For this review, take the finished solid that the model builds, in its own axes (mm). Face numbers are marked on the shaded views. A direction names the side the tool comes from. Coordinates: 2 decimals unless noted, no trailing zeros. Write each loop counter-clockwise with the first axis right and the second up, starting at its lowest first coordinate (ties: lowest second). Pieces come first, ordered by that corner, then holes. Notation, with made-up numbers: (72.25, 67.25) -> (115.25, 67.25) arc R17 ccw to (115.25, 84.25) -> close; hole circle Ø10 at (26.5, 21.25). An arc over 180 degrees is marked (long way). One line per item, written item: value. Start each with the question number.
1) Mouldability with a two-part tool opening along Z and no side actions: class the marked faces 3, 4 and 5 as released by +Z, released by -Z, zero draft, split by the parting line, or undercut.
2) Add section A-A (x = -10). State the section outline as (y, z) points.
3) Add section B-B (y = 15). State the section outline as (x, z) points.
4) For probe 1 along Y at (x, z) = (-20, 24.25); probe 2 along Z at (x, y) = (-3, 53); probe 3 along X at (y, z) = (41.5, 4.5), list the stretches that pass through material, from the lowest coordinate up. Write a range as from..to.
5) Add section D-D (y = 5.5). State the section outline as (x, z) points, and give its area (3 significant figures).
6) For pin 1 Ø6 at (x, z) = (-5, 19.5) entering from +Y; pin 2 Ø2 at (y, z) = (64.5, -8.5) entering from +X, all flat-tipped, find the tip position at first contact; note any pin that passes through.
7) Add section C-C (x = -20). State the section outline as (y, z) points, and give its area (3 significant figures).
8) Machinability: for the marked faces 1 and 2, which of the approach directions +Z, -Z, +X, -X, +Y, -Y give a long, thin tool a straight path to every point of the face, cutting with its end or side? Answer none if there is none.
from build123d import *

# Parameters (mm, degrees)
SKETCH_1_W          = 74
SKETCH_1_H          = 44
EXTRUDE_1_DEPTH     = 80
SKETCH_2_W          = 41.146480438
SKETCH_2_H          = 58.393385187
CUT_EXTRUDE_1_DEPTH = 81
SKETCH_3_R          = 4.05
CUT_EXTRUDE_2_DEPTH = 51


with BuildPart() as part:
    # Эскиз1 → Вытянуть-Тонкостенный1 (new body)
    with BuildSketch(Plane(origin=(0, 0, 0), x_dir=(1, 0, 0), z_dir=(0, 1, 0))):
        with BuildLine():
            Line((40, 22), (40, -22))
            ThreePointArc((40, -22), (39.121320344, -24.121320344), (37, -25))
            Line((37, -25), (-37, -25))
            ThreePointArc((-37, -25), (-39.121320344, -24.121320344), (-40, -22))
            Line((-40, -22), (-40, 22))
            ThreePointArc((-40, 22), (-39.121320344, 24.121320344), (-37, 25))
            Line((-37, 25), (37, 25))
            ThreePointArc((37, 25), (39.121320344, 24.121320344), (40, 22))
        make_face()
        Rectangle(SKETCH_1_W, SKETCH_1_H, mode=Mode.SUBTRACT)
    extrude(amount=EXTRUDE_1_DEPTH)

    # Эскиз2 → Вырез-Вытянуть1 (cut, through all)
    with BuildSketch(Plane(origin=(0, 80, 0), x_dir=(1, 0, 0), z_dir=(0, 1, 0))):
        with Locations((20.573240219, 1.776081122)):
            Rectangle(SKETCH_2_W, SKETCH_2_H)
    extrude(amount=-CUT_EXTRUDE_1_DEPTH, mode=Mode.SUBTRACT)

    # Эскиз3 → Вырез-Вытянуть2 (cut, through all)
    with BuildSketch(Plane(origin=(0, 0, -25), x_dir=(-1, 0, 0), z_dir=(0, 0, -1))):
        with Locations((20, 115)):
            Circle(SKETCH_3_R)
        with Locations((20, 15)):
            Circle(SKETCH_3_R)
        with Locations((20, 65)):
            Circle(SKETCH_3_R)
    extrude(amount=-CUT_EXTRUDE_2_DEPTH, mode=Mode.SUBTRACT)


solid = part.part
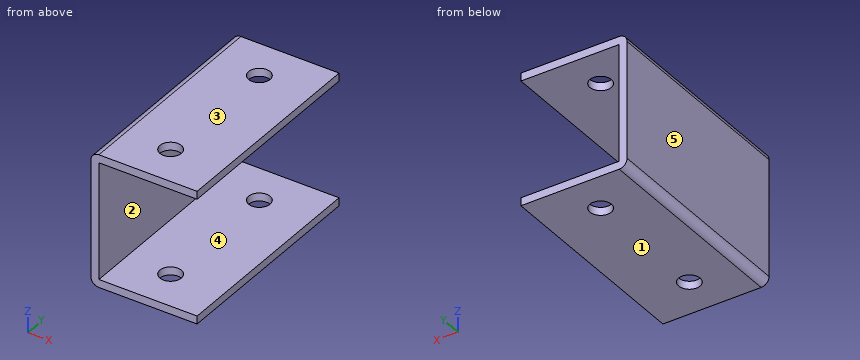
Numbers:
1. face 3: released by +Z
1. face 4: undercut
1. face 5: zero draft
2. outline: (0, -25) -> (80, -25) -> (80, -22) -> (0, -22) -> close; (0, 22) -> (80, 22) -> (80, 25) -> (0, 25) -> close
3. outline: (-40, -22) arc R3 ccw to (-37, -25) -> (-24.05, -25) -> (-24.05, -22) -> (-37, -22) -> (-37, 22) -> (-24.05, 22) -> (-24.05, 25) -> (-37, 25) arc R3 ccw to (-40, 22) -> close; (-15.95, -25) -> (0, -25) -> (0, -22) -> (-15.95, -22) -> close; (-15.95, 22) -> (0, 22) -> (0, 25) -> (-15.95, 25) -> close
4. probe 1: 0..10.95, 19.05..60.95, 69.05..80
4. probe 2: -25..-22, 22..25
4. probe 3: -40..-37
5. outline: (-40, -22) arc R3 ccw to (-37, -25) -> (0, -25) -> (0, -22) -> (-37, -22) -> (-37, 22) -> (0, 22) -> (0, 25) -> (-37, 25) arc R3 ccw to (-40, 22) -> close
5. area: 368 mm²
6. pin 1: y = 80
6. pin 2: x = -37
7. outline: (0, -25) -> (10.95, -25) -> (10.95, -22) -> (0, -22) -> close; (0, 22) -> (10.95, 22) -> (10.95, 25) -> (0, 25) -> close; (19.05, -25) -> (60.95, -25) -> (60.95, -22) -> (19.05, -22) -> close; (19.05, 22) -> (60.95, 22) -> (60.95, 25) -> (19.05, 25) -> close; (69.05, -25) -> (80, -25) -> (80, -22) -> (69.05, -22) -> close; (69.05, 22) -> (80, 22) -> (80, 25) -> (69.05, 25) -> close
7. area: 383 mm²
8. face 1: -Z, +X, -X, +Y, -Y
8. face 2: +X, +Y, -Y
